Here's how the part is built. I have some questions about the finished solid (model axes, mm). Face numbers are marked on the shaded views. A direction names the side the tool comes from. Coordinates: 2 decimals unless noted, no trailing zeros. Write each loop counter-clockwise with the first axis right and the second up, starting at its lowest first coordinate (ties: lowest second). Pieces come first, ordered by that corner, then holes. Notation, with made-up numbers: M -15,-15 L 40,-15 A26 ccw 40,22 Z; hole C -6,62.5 d7. An arc over 180 degrees is marked long. Use a Markdown table: item, result.
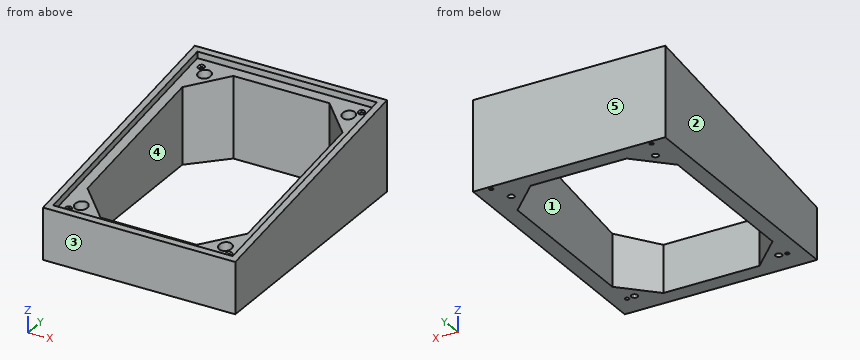
```python
from build123d import *

# Parameters (mm, degrees)
F0_W           = 150
F0_H           = 200
F0_W_2         = 137.5
F0_H_2         = 187.5
F0_R           = 5
F1_DEPTH       = 70
F3_DEPTH       = 155
F5_START       = -5
F5_DEPTH       = 140
F0_R_2         = 2.5
F6_DEPTH       = 5
F8_D           = 3
F8_CSINK_D     = 5
F8_CSINK_ANGLE = 90


with BuildPart() as f1:
    # F0 (on Top) → F1 (new body)
    with BuildSketch(Plane.XY):
        with Locations((0.0049619689, -0.0823242008)):
            Rectangle(F0_W, F0_H)
        with Locations((0.0049619689, -0.0823242008)):
            Rectangle(F0_W_2, F0_H_2, mode=Mode.SUBTRACT)
        with Locations((0.0049619689, -0.0823242008)):
            Rectangle(F0_W_2, F0_H_2)
        Polygon((-62.4950380311, 62.4176757992), (-62.4950380311, 87.4176757992), (-37.4950380311, 87.4176757992), (37.5049619689, 87.4176757992), (62.5049619689, 87.4176757992), (62.5049619689, 62.4176757992), (62.5049619689, -62.5823242008), (62.5049619689, -87.5823242008), (37.5049619689, -87.5823242008), (-37.4950380311, -87.5823242008), (-62.4950380311, -87.5823242008), (-62.4950380311, -62.5823242008), align=None, mode=Mode.SUBTRACT)
        Polygon((-37.4950380311, 87.4176757992), (-62.4950380311, 87.4176757992), (-62.4950380311, 62.4176757992), align=None)
        with Locations((-56.2450380311, 81.1676757992)):
            Circle(F0_R, mode=Mode.SUBTRACT)
        Polygon((62.5049619689, 87.4176757992), (37.5049619689, 87.4176757992), (62.5049619689, 62.4176757992), align=None)
        with Locations((56.2549619689, 81.1676757992)):
            Circle(F0_R, mode=Mode.SUBTRACT)
        Polygon((62.5049619689, -87.5823242008), (62.5049619689, -62.5823242008), (37.5049619689, -87.5823242008), align=None)
        with Locations((56.2549619689, -81.3323242008)):
            Circle(F0_R, mode=Mode.SUBTRACT)
        Polygon((-37.4950380311, -87.5823242008), (-62.4950380311, -62.5823242008), (-62.4950380311, -87.5823242008), align=None)
        with Locations((-56.2450380311, -81.3323242008)):
            Circle(F0_R, mode=Mode.SUBTRACT)
    extrude(amount=F1_DEPTH)

    # F2 (on face) → F3 (cut)
    with BuildSketch(Plane.YZ.offset(75.0049619689)):
        Polygon((-100.0823242008, 70), (-100.0823242008, 40), (99.9176757992, 70), align=None)
    extrude(amount=-F3_DEPTH, mode=Mode.SUBTRACT)

    # F4 (on face) → F5 (cut)
    with BuildSketch(Plane.YZ.offset(75.0049619689).offset(F5_START)):
        Polygon((94.9176757992, 69.25), (-95.0823242008, 40.75), (-95.0823242008, 35.75), (94.9176757992, 64.25), align=None)
    extrude(amount=-F5_DEPTH, mode=Mode.SUBTRACT)

    # F0 (on Top) → F6 (join)
    with BuildSketch(Plane.XY):
        with Locations((-56.2450380311, 81.1676757992)):
            Circle(F0_R)
        with Locations((-56.2450380311, 81.1676757992)):
            Circle(F0_R_2, mode=Mode.SUBTRACT)
        with Locations((56.2549619689, 81.1676757992)):
            Circle(F0_R)
        with Locations((56.2549619689, 81.1676757992)):
            Circle(F0_R_2, mode=Mode.SUBTRACT)
        with Locations((-56.2450380311, -81.3323242008)):
            Circle(F0_R)
        with Locations((-56.2450380311, -81.3323242008)):
            Circle(F0_R_2, mode=Mode.SUBTRACT)
        with Locations((56.2549619689, -81.3323242008)):
            Circle(F0_R)
        with Locations((56.2549619689, -81.3323242008)):
            Circle(F0_R_2, mode=Mode.SUBTRACT)
    extrude(amount=F6_DEPTH)

    # F8 (through all)
    with Locations(Plane(origin=(0, -7.3367748602, 48.9118324011), x_dir=(1, 0, 0), z_dir=(0, -0.1483404529, 0.9889363529))):
        with Locations((-62.4950380311, 95.8145085723), (62.5049619689, 95.8145085723), (62.5049619689, -81.143290069), (-62.4950380311, -81.143290069)):
            CounterSinkHole(F8_D / 2, F8_CSINK_D / 2, counter_sink_angle=F8_CSINK_ANGLE)


solid = f1.part
```
1. I need wall thicknesses on probe 1 along X at (y, z) = (-29.5, 33); probe 2 along Y at (x, z) = (16, 16); probe 3 along X at (y, z) = (68, 62.5). Which ranges of each line are inside material? Lowest first, please.
Answers follow:
| item | result |
|---|---|
| probe 1 | x = -75 to -62.5, 62.5 to 75 |
| probe 2 | y = -100.08 to -87.58, 87.42 to 99.92 |
| probe 3 | x = -75 to -70, 70 to 75 |
2. We'd pull the mould along Y, two halves only. Please class the marked faces 1, 2 and 3: +Y half, -Y half, draft (parallel to the pull), parting line (faces both ways), or undercut.
Answers follow:
| item | result |
|---|---|
| face 1 | undercut |
| face 2 | draft |
| face 3 | -Y half |
3. Suppose I cut it at A-A on y = 23.5. Write out the boundary of the cut face in (x, z).
Answers follow:
| item | result |
|---|---|
| outline | M -75,0 L -62.5,0 L -62.5,53.54 L -70,53.54 L -70,58.54 L -75,58.54 Z; M 62.5,0 L 75,0 L 75,58.54 L 70,58.54 L 70,53.54 L 62.5,53.54 Z |
4. Suppose I cut it at C-C on z = 21.5. State how many separate pieces and enclosed holes the cut face has, and give its area (3 significant figures).
Answers follow:
| item | result |
|---|---|
| separate pieces | 1 |
| enclosed holes | 9 |
| area | 9,030 mm2 |
5. Will these pins go through, and if not, where does the flat tip stop? pin 1 Ø3 at (x, y) = (57.5, -80.5) entering from +Z; pin 2 Ø1.5 at (x, z) = (20.5, 67.5) entering from -Y.
Answers follow:
| item | result |
|---|---|
| pin 1 | stops at z = 5 |
| pin 2 | stops at y = 94.92 |
6. Suppose I cut it at B-B on x = -29. Write out the boundary of the cut face in (y, z) (3 decimals).
Answers follow:
| item | result |
|---|---|
| outline | M -100.082,0 L -87.582,0 L -87.582,36.875 L -95.082,35.75 L -95.082,40.75 L -100.082,40 Z; M 87.418,0 L 99.918,0 L 99.918,70 L 94.918,69.25 L 94.918,64.25 L 87.418,63.125 Z |
7. Which directions (+Z, -Z, +X, -X, +Y, -Y) give clear straight access to the entire face, cutting with the end or side of a thin tool? Please do the marked faces 4 and 5.
Answers follow:
| item | result |
|---|---|
| face 4 | +Z, -Z |
| face 5 | +Z, -Z, +X, -X, +Y |
